Source: CAD feature listing. Evaluate the final solid. Frame: model axes, mm. Face numbers are marked on the shaded views. A direction names the side the tool comes from. Round coordinates to 2 decimals unless told otherwise and drop trailing zeros. Order: outer loops, then holes, each group sorted by start corner. A loop starts at its lowest first (then second) coordinate and runs counter-clockwise, first axis right, second up. Notation, with made-up numbers: (0, -24.75) -> (21, -24.75) arc R35 cw to (21, 12.25) -> close; hole circle Ø2 at (74.25, 22.25). An arc over 180 degrees is marked (long way). Answer as CSV lines item,"result". Start each with the question number.
(1) Section query A-A (z = -10). Output: boundary loops of the cut face in (x, y).
(2) Set-up query: the marked faces 1, 2 and 3. Return all of +Z, -Z, +X, -X, +Y, -Y with unobstructed straight access to the full face (end or side cutting, diameter ignored); none if empty.
(3) Section query D-D (x = 14). Output: boundary loops of the cut face in (y, z).
(4) Line query: line 1 along X through (y, z) = (29.5, -9); line 2 along Y through (x, z) = (39.5, 11.5); line 3 along X through (y, z) = (4.5, 12). Output: solid intervals per line, ascending. Write a range as from..to.
(5) Contact query for flat-ended pins moving along their axis: P1, Ø11, axis at x = 37.5, y = 34.5, coming from the +Z side; P2, Ø11, axis at x = 38.5, y = 10.5, coming from the -Z side; P3, Ø12, axis at y = 26, z = -11, coming from the +X side; P4, Ø1, axis at x = -15.5, y = 25.5, coming from the +Z side. Output: stop coordinate, or through.
(6) Section query C-C (y = 5.5). Output: boundary loops of the cut face in (x, z), plus the area to 3 significant figures.
(7) Section query B-B (x = 4). Output: boundary loops of the cut face in (y, z), plus the area to 3 significant figures.
```python
from build123d import *

# Parameters (mm, degrees)
BOSS_EXTRUDE1_DEPTH = 40
SKETCH2_R           = 2.5
CUT_EXTRUDE1_DEPTH  = 97.046863561
CUT_EXTRUDE2_REACH  = 91.123
SKETCH3_R           = 7.625
SKETCH4_R           = 4.5
CUT_EXTRUDE4_DEPTH  = 10
SKETCH4_4_W         = 10
SKETCH4_4_H         = 16.5
BOSS_EXTRUDE2_DEPTH = 10
CUT_EXTRUDE5_REACH  = 101.027
SKETCH2_3_R         = 2.25


with BuildPart() as part:
    # Sketch1 → Boss-Extrude1 (new body)
    with BuildSketch(Plane(origin=(0, 0, 0), x_dir=(1, 0, 0), z_dir=(0, 1, 0))):
        Polygon((-35, -42.269292904), (-30, -42.269292904), (-30, 32.730707096), (30, 32.730707096), (30, -42.269292904), (32.5, -42.269292904), (32.5, 37.730707096), (-35, 37.730707096), align=None)
    extrude(amount=BOSS_EXTRUDE1_DEPTH)

    # Sketch2 → Cut-Extrude1 (cut, through all)
    with BuildSketch(Plane(origin=(0, 0, -37.730707096), x_dir=(-1, 0, 0), z_dir=(0, 0, -1))):
        with Locations((5.1985867, 23.03894843)):
            Circle(SKETCH2_R)
        with Locations((0.002434277, 14.03894843)):
            Circle(SKETCH2_R)
        with Locations((-5.193718146, 23.03894843)):
            Circle(SKETCH2_R)
    extrude(amount=-CUT_EXTRUDE1_DEPTH, mode=Mode.SUBTRACT)

    # Sketch3 → Cut-Extrude2 (cut, up to next)
    with BuildSketch(Plane.ZY.offset(35), mode=Mode.PRIVATE) as cut_extrude2_sk1:
        with Locations((27.269292904, 20)):
            Circle(SKETCH3_R)
    cut_extrude2_tool1 = extrude(cut_extrude2_sk1.sketch, amount=-CUT_EXTRUDE2_REACH, mode=Mode.PRIVATE) & part.part
    add(cut_extrude2_tool1.solids().sort_by_distance((-35, 20, 27.269293))[0], mode=Mode.SUBTRACT)

    # Sketch4 → Cut-Extrude4 (cut)
    with BuildSketch(Plane(origin=(32.5, 0, 0), x_dir=(0, 0, -1), z_dir=(1, 0, 0))):
        with Locations((-27.269292904, 20)):
            Circle(SKETCH4_R)
    extrude(amount=-CUT_EXTRUDE4_DEPTH, mode=Mode.SUBTRACT)

    # Sketch4<4> → Boss-Extrude2 (add)
    with BuildSketch(Plane(origin=(32.5, 0, 0), x_dir=(0, 0, -1), z_dir=(1, 0, 0))):
        with Locations((-12.269292904, 8.25)):
            Rectangle(SKETCH4_4_W, SKETCH4_4_H)
        with Locations((-12.269292904, 31.75)):
            Rectangle(SKETCH4_4_W, SKETCH4_4_H)
    extrude(amount=BOSS_EXTRUDE2_DEPTH)

    # Sketch2<3> → Cut-Extrude5 (cut, up to next)
    with BuildSketch(Plane(origin=(0, 0, -37.730707096), x_dir=(-1, 0, 0), z_dir=(0, 0, -1)), mode=Mode.PRIVATE) as cut_extrude5_sk1:
        with Locations((0.002434277, 20.03894843)):
            Circle(SKETCH2_3_R)
    cut_extrude5_tool1 = extrude(cut_extrude5_sk1.sketch, amount=-CUT_EXTRUDE5_REACH, mode=Mode.PRIVATE) & part.part
    add(cut_extrude5_tool1.solids().sort_by_distance((-0.002434, 20.038948, -37.730707))[0], mode=Mode.SUBTRACT)


solid = part.part
```
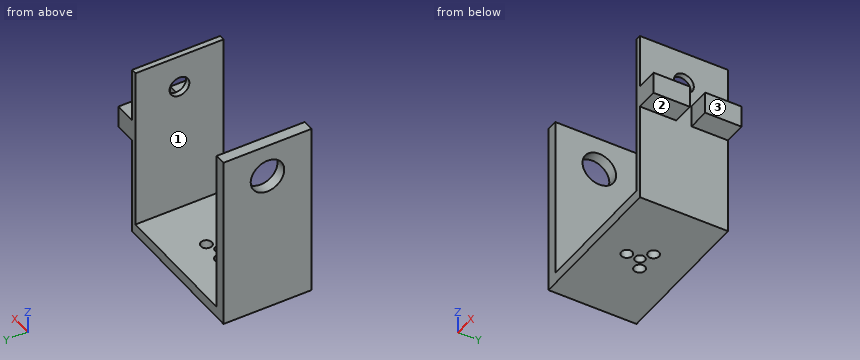
Answer block:
1,outline,"(-35, 0) -> (-30, 0) -> (-30, 40) -> (-35, 40) -> close; (30, 0) -> (32.5, 0) -> (32.5, 40) -> (30, 40) -> close"
2,face 1,"+Z, +Y, -Y"
2,face 2,"-Z, +X, +Y, -Y"
2,face 3,"+Z, -Z, +X, +Y, -Y"
3,outline,"(0, -37.73) -> (40, -37.73) -> (40, -32.73) -> (0, -32.73) -> close"
4,line 1,"-35..-30, 30..32.5"
4,line 2,"0..16.5, 23.5..40"
4,line 3,"-35..-30, 30..42.5"
5,P1,"z = 42.27"
5,P2,"z = 7.27"
5,P3,"x = 32.5"
5,P4,"z = -32.73"
6,outline,"(-35, -37.73) -> (32.5, -37.73) -> (32.5, 7.27) -> (42.5, 7.27) -> (42.5, 17.27) -> (32.5, 17.27) -> (32.5, 42.27) -> (30, 42.27) -> (30, -32.73) -> (-30, -32.73) -> (-30, 42.27) -> (-35, 42.27) -> close"
6,area,"1,000 mm2"
7,outline,"(0, -37.73) -> (20.84, -37.73) -> (20.84, -32.73) -> (0, -32.73) -> close; (25.24, -37.73) -> (40, -37.73) -> (40, -32.73) -> (25.24, -32.73) -> close"
7,area,"178 mm2"
